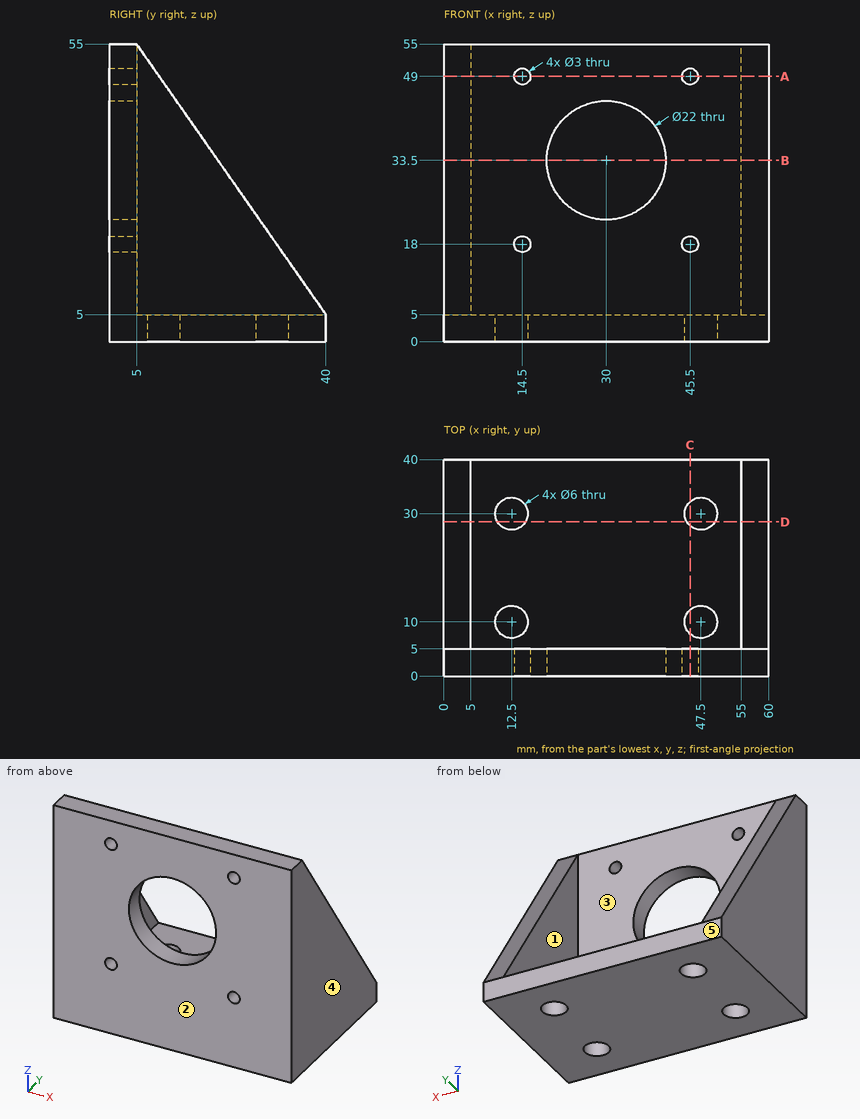
Answer from the drawing. Dimensions are ordinates in mm from the lowest x, y and z of the part. A direction names the side the tool comes from. Round coordinates to 2 decimals unless told otherwise and drop trailing zeros. Loops run counter-clockwise (first coordinate to the right, second up) from the corner with the lowest first, then second, coordinate; pieces in that order, holes last. Notation, with made-up numbers: (8.25, -32) - (49.25, -32) arc R28 cw to (49.25, 4) - close; hole circle Ø9 at (70.25, 76). An arc over 180 degrees is marked (long way). Return JSON: item names as keys, results as strings. Group by question number.
1. The part is cut by section A-A on z = 49. Determine the outline of the cut face in (x, y), then the cut area to 3 significant figures.
2. The part is cut by section B-B on z = 33.5. Determine the outline of the cut face in (x, y).
3. Which of the six approach directions +Z, -Z, +X, -X, +Y, -Y give full straight-line access (tool end or side, diameter ignored) to the marked faces 1 and 2?
4. Consider probe 1 along X at (y, z) = (3, 18); probe 2 along Y at (x, z) = (12.5, 1.2); probe 3 along X at (y, z) = (6, 8). Determine where each line is inside the solid, lowest interval first.
5. The part is cut by section D-D on y = 28.5. Determine the outline of the cut face in (x, z).
6. Each of these flat-tipped pins is pushed along its axis until it touches: P1, Ø12, axis at x = 48, z = 21.5, coming from the +Y side; P2, Ø2.5, axis at x = 45.5, z = 18, coming from the -Y side; P3, Ø17.5, axis at x = 21.5, y = 31, coming from the +Z side. Where does it stop, or does it pass through?
7. The part is cut by section C-C on x = 45.5. Determine the outline of the cut face in (y, z), then the cut area to 3 significant figures.
8. The mould has two halves that part along X. Classify the marked faces 3, 4 and 5: pulls with the +X half, pulls with the -X half, needs draft (parallel to the pull), parting line crosses it, or undercut.
Resolved:
{
 "1": {"outline": "(0, 0) - (13, 0) - (13, 5) - (5, 5) - (5, 9.2) - (0, 9.2) - close; (16, 0) - (44, 0) - (44, 5) - (16, 5) - close; (47, 0) - (60, 0) - (60, 9.2) - (55, 9.2) - (55, 5) - (47, 5) - close", "area": "312 mm²"},
 "2": {"outline": "(0, 0) - (19, 0) - (19, 5) - (5, 5) - (5, 20.05) - (0, 20.05) - close; (41, 0) - (60, 0) - (60, 20.05) - (55, 20.05) - (55, 5) - (41, 5) - close"},
 "3": {"face 1": "+Z, +Y", "face 2": "+Z, -Z, +X, -X, -Y"},
 "4": {"probe 1": "x = 0 to 13, 16 to 44, 47 to 60", "probe 2": "y = 0 to 7, 13 to 27, 33 to 40", "probe 3": "x = 0 to 5, 55 to 60"},
 "5": {"outline": "(0, 0) - (9.9, 0) - (9.9, 5) - (5, 5) - (5, 21.43) - (0, 21.43) - close; (15.1, 0) - (44.9, 0) - (44.9, 5) - (15.1, 5) - close; (50.1, 0) - (60, 0) - (60, 21.43) - (55, 21.43) - (55, 5) - (50.1, 5) - close"},
 "6": {"P1": "stops at y = 5", "P2": "passes through", "P3": "stops at z = 5"},
 "7": {"outline": "(0, 0) - (7.76, 0) - (7.76, 5) - (5, 5) - (5, 16.5) - (0, 16.5) - close; (0, 19.5) - (5, 19.5) - (5, 47.5) - (0, 47.5) - close; (0, 50.5) - (5, 50.5) - (5, 55) - (0, 55) - close; (12.24, 0) - (27.76, 0) - (27.76, 5) - (12.24, 5) - close; (32.24, 0) - (40, 0) - (40, 5) - (32.24, 5) - close", "area": "375 mm²"},
 "8": {"face 3": "undercut", "face 4": "pulls with the +X half", "face 5": "needs draft"}
}
